Input: part model. Units: mm. Frame: model coordinates. Round coordinates to 2 decimals unless told otherwise and drop trailing zeros. Loops run counter-clockwise (first coordinate to the right, second up) from the corner with the lowest first, then second, coordinate; pieces in that order, holes last.
(1) Cut plane A-A, the plane z = 0. Output: boundary loops of the cut face in (x, y).
(2) Draft query along X for faces 1 (the face through (0.867, 0.035, -3.905)), 2 (the face through (-10, 0, 1)), 3 (the face through (4.3, -2.5, 1)), 4 (the face through (10, 0, 1)). Return one class per face: released by +X, released by -X, zero draft, split by the parting line, or undercut.
(3) Cut plane C-C, the plane y = 1. Output: boundary loops of the cut face in (x, z), and give its area (3 significant figures).
(4) Line query: line 1 (Z direction, x = -0.25, y = 1.5); line 2 (Z direction, x = 1.25, y = -1.4). Output: solid intervals per line, ascending.
(5) Cut plane B-B, the plane x = 0. Output: boundary loops of the cut face in (y, z), and give its area (3 significant figures).
from build123d import *

# Parameters (mm, degrees)
SKETCH1_W                       = 20
SKETCH1_H                       = 5
BOSS_EXTRUDE1_DEPTH             = 106
SKETCH2_R                       = 4
HOLES_FOR_20MM_STRIP_ONLY_DEPTH = 107.587991819
SKETCH5_OUTSIDE_W               = 64.6
SKETCH5_OUTSIDE_H               = 256.6
SKETCH5_OUTSIDE_W_2             = 51.505008444
SKETCH5_OUTSIDE_H_2             = 150
CUT_EXTRUDE3_DEPTH              = 107.587991819


with BuildPart() as part:
    # Sketch1 → Boss-Extrude1 (new, symmetric)
    with BuildSketch(Plane.XY):
        Rectangle(SKETCH1_W, SKETCH1_H)
    extrude(amount=BOSS_EXTRUDE1_DEPTH, both=True)

    # Sketch2 → Holes for 20mm strip ONLY (cut, through all)
    with BuildSketch(Plane(origin=(0, 2.5, 0), x_dir=(1, 0, 0), z_dir=(0, 1, 0))):
        with Locations(Location((0, 87.5, 0), (0, 0, 180))):
            Circle(SKETCH2_R)
        with Locations(Location((0, 0, 0), (0, 0, 180))):
            Circle(SKETCH2_R)
        with Locations(Location((0, -87.5, 0), (0, 0, 180))):
            Circle(SKETCH2_R)
    extrude(amount=-HOLES_FOR_20MM_STRIP_ONLY_DEPTH, mode=Mode.SUBTRACT)

    # Sketch5 outside → Cut-Extrude3 (cut, through all)
    with BuildSketch(Plane(origin=(0, 2.5, 0), x_dir=(1, 0, 0), z_dir=(0, 1, 0))):
        Rectangle(SKETCH5_OUTSIDE_W, SKETCH5_OUTSIDE_H)
        Rectangle(SKETCH5_OUTSIDE_W_2, SKETCH5_OUTSIDE_H_2, mode=Mode.SUBTRACT)
    extrude(amount=-CUT_EXTRUDE3_DEPTH, mode=Mode.SUBTRACT)


solid = part.part
Reported:
1. outline: (-10, -2.5) - (-4, -2.5) - (-4, 2.5) - (-10, 2.5) - close; (4, -2.5) - (10, -2.5) - (10, 2.5) - (4, 2.5) - close
2. face 1: undercut
2. face 2: released by -X
2. face 3: zero draft
2. face 4: released by +X
3. outline: (-10, -75) - (10, -75) - (10, 75) - (-10, 75) - close; hole circle Ø8 at (0, 0)
3. area: 2,950 mm2
4. line 1: z = -75 to -3.99, 3.99 to 75
4. line 2: z = -75 to -3.8, 3.8 to 75
5. outline: (-2.5, -75) - (2.5, -75) - (2.5, -4) - (-2.5, -4) - close; (-2.5, 4) - (2.5, 4) - (2.5, 75) - (-2.5, 75) - close
5. area: 710 mm2
